Autodesk Inventor part; units mm, degrees
ref_plane "YZ Plane" through (0, 0, 0) normal (1, 0, 0) x (0, 1, 0)
ref_plane "XZ Plane" through (0, 0, 0) normal (0, 1, 0) x (-1, 0, 0)
ref_plane "XY Plane" through (0, 0, 0) normal (0, 0, 1) x (1, 0, 0)
sketch "スケッチ1" plane through (0, 0, 0) normal (0, 1, 0) x (-1, 0, 0)
  line L0 (-27.5, -9.5) -> (27.5, -9.5)
  line L1 (27.5, -9.5) -> (27.5, 9.5)
  line L2 (27.5, 9.5) -> (-27.5, 9.5)
  line L3 (-27.5, 9.5) -> (-27.5, -9.5)
  line L4 (-27.5, -9.5) -> (27.5, 9.5) construction
  line L5 (27.5, -9.5) -> (-27.5, 9.5) construction
  point P0 (0, 0)
  dimension "d0" = 19
  dimension "d1" = 55
extrude "プレート1" add sketch "スケッチ1" along normal blind 2
sketch "スケッチ2" plane through (27.5, 0, 9.5) normal (1, 0, 0) x (0, 0, -1)
  line L0 (0, 2) -> (19, 2)
  line L1 (19, 2) -> (0, 2)
  line L2 (0, 2) -> (0, 22)
  line L3 (0, 22) -> (19, 22)
  line L4 (19, 22) -> (19, 2)
  point P0 (9.5, 0)
  dimension "d3" = 20
sheet face with bend "面2" sketch "スケッチ2" thickness 2 toward (1, 0, 0) bend radius 2
bend "曲げ1"
sketch "スケッチ3" plane through (-27.5, 0, -9.5) normal (-1, 0, 0) x (0, 0, 1)
  line L0 (0, 0) -> (0, 2)
  line L1 (0, 22) -> (19, 22)
  line L2 (0, 2) -> (19, 2)
  line L3 (19, 2) -> (19, 22)
  line L4 (19, 22) -> (0, 22)
  line L5 (0, 22) -> (0, 2)
  point P0 (9.5, 0)
sheet face with bend "面3" sketch "スケッチ3" thickness 2 toward (-1, 0, 0) bend radius 2
bend "曲げ2"
sketch "スケッチ4" plane through (-29.5, 0, -9.5) normal (-1, 0, 0) x (0, 0, 1)
  line L0 (7.5, 18) -> (7.5, 8)
  arc A0 (7.5, 8) -> (11.5, 8) centre (9.5, 8) ccw
  line L1 (11.5, 8) -> (11.5, 18)
  arc A1 (11.5, 18) -> (7.5, 18) centre (9.5, 18) ccw
  line L2 (19, 22) -> (19, 4)
  line L3 (0, 22) -> (19, 22)
  line L4 (19, 4) -> (0, 4)
  point P0 (9.5, 0)
  dimension "d18" = 2
  dimension "d33" = 4
  dimension "d34" = 4
extrude "押し出し1" cut sketch "スケッチ4" against normal blind 100
sketch "スケッチ5" plane through (0, 2, 0) normal (0, 1, 0) x (1, 0, 0)
  line L0 (-19.5, -2) -> (19.5, -2)
  arc A0 (19.5, -2) -> (19.5, 2) centre (19.5, 0) ccw
  line L1 (19.5, 2) -> (-19.5, 2)
  arc A1 (-19.5, 2) -> (-19.5, -2) centre (-19.5, 0) ccw
  line L2 (25.5, -9.5) -> (-25.5, -9.5)
  line L3 (-25.5, 9.5) -> (-25.5, -9.5)
  line L4 (25.5, -9.5) -> (25.5, 9.5)
  point P0 (0, 0)
  point P1 (-21.5, 0)
  dimension "d22" = 2
  dimension "d35" = 6
  dimension "d36" = 6
extrude "押し出し2" cut sketch "スケッチ5" against normal blind 3
equation "\"d2\" = Thickness"
equation "\"d4\" = BendRadius"
equation "\"d5\" = BendReliefWidth"
equation "\"d7\" = MinimumRemnant"
equation "\"d6\" = BendReliefDepth"
equation "\"d8\" = TransitionRadius"
equation "\"d9\" = BendRadius"
equation "\"d10\" = BendReliefWidth"
equation "\"d12\" = MinimumRemnant"
equation "\"d11\" = BendReliefDepth"
equation "\"d13\" = TransitionRadius"
equation "\"BendRadius\" = Thickness"
equation "\"BendReliefWidth\" = Thickness"
equation "\"BendReliefDepth\" = 0.5 * Thickness"
equation "\"CornerReliefSize\" = 4 * Thickness"
equation "\"MinimumRemnant\" = 2 * Thickness"
equation "\"TransitionRadius\" = BendRadius"
equation "\"JacobiRadiusSize\" = BendRadius"
equation "\"GapSize\" = Thickness"
properties part number "thumbkey_cup" material "アルミニウム 6061"
The model under review builds one solid part; all positions refer to its coordinate system, in mm. A direction names the side the tool comes from. Give positions to 0.01 mm unless a question says otherwise; leave off trailing zeros. Write each loop counter-clockwise with the first axis right and the second up, starting at its lowest first coordinate (ties: lowest second). Pieces come first, ordered by that corner, then holes. Notation, with made-up numbers: (23.25, 66.5) - (38.25, 66.5) arc R19 cw to (38.25, 76.5) - close; hole circle Ø3 at (67.25, -36). An arc over 180 degrees is marked (long way). Answer in a Markdown table with one row per item. Add a question column.
1. Draft analysis for pull direction Y (two halves, no side actions). For faces 1 (the flat face through (0, 1, 2)), 2 (the cylindrical face through (28, 20, 0)), 3 (the flat face through (28, 22, 0)), 4 (the cylindrical face through (28, 6, 0)), state which applies: +Y half, -Y half, draft (parallel to the pull), parting line (faces both ways), or undercut.
2. Wall thickness on line 1 along X through (y, z) = (6, 4.25); line 2 along Y through (x, z) = (-22.5, -4.5); line 3 along X through (y, z) = (2.75, 3.5): over which ranges is each line inside the solid? List them lowest first. Write a range as [from, to].
3. We need section D-D on y = 17. Write out the cut boundary in (x, z).
4. We need section B-B on z = 0. Write out the cut boundary in (x, y), then the cut area to 3 significant figures.
5. Tool access review of faces 5 (the flat face through (0.1, 0.4, -9.5)), 6 (the cylindrical face through (-21.5, 1, 0)), 7 (the cylindrical face through (-29, 6, 0)), 8 (the cylindrical face through (26.93, 2.6, -0.13)): name each direction out of +Z, -Z, +X, -X, +Y, -Y from which nothing blocks a thin tool from reaching the whole face with its end or side.
6. We need section C-C on x = 3.5. Write out the cut boundary in (y, z).
7. We need section A-A on y = 4.75. Write out the cut boundary in (x, z), then the cut area to 3 significant figures.
8. Insertion check: P1, Ø3, axis at x = -14, z = -2.5, coming from the +Y side; P2, Ø9, axis at y = 10.5, z = -1, coming from the +X side. Each pin has a flat end and moves straight along its axis. Give the tip position at first contact, or say it passes through.
Ans:
| question | item | result |
|---|---|---|
| 1 | face 1 | draft |
| 1 | face 2 | undercut |
| 1 | face 3 | +Y half |
| 1 | face 4 | undercut |
| 2 | line 1 | x = [-29.5, -27.5], [27.5, 29.5] |
| 2 | line 2 | y = [0, 2] |
| 2 | line 3 | x = [-29.3, -27.06], [27.06, 29.3] |
| 3 | outline | (-29.5, -9.5) - (-27.5, -9.5) - (-27.5, -2) - (-29.5, -2) - close; (-29.5, 2) - (-27.5, 2) - (-27.5, 9.5) - (-29.5, 9.5) - close; (27.5, -9.5) - (29.5, -9.5) - (29.5, -2) - (27.5, -2) - close; (27.5, 2) - (29.5, 2) - (29.5, 9.5) - (27.5, 9.5) - close |
| 4 | outline | (-29.5, 4) arc R4 ccw to (-25.5, 0) - (-21.5, 0) - (-21.5, 2) - (-25.5, 2) arc R2 cw to (-27.5, 4) - (-27.5, 6) - (-29.5, 6) - close; (-29.5, 20) - (-27.5, 20) - (-27.5, 22) - (-29.5, 22) - close; (21.5, 0) - (25.5, 0) arc R4 ccw to (29.5, 4) - (29.5, 6) - (27.5, 6) - (27.5, 4) arc R2 cw to (25.5, 2) - (21.5, 2) - close; (27.5, 20) - (29.5, 20) - (29.5, 22) - (27.5, 22) - close |
| 4 | area | 50.8 mm^2 |
| 5 | face 5 | -Z, +X, -X, +Y, -Y |
| 5 | face 6 | +Y, -Y |
| 5 | face 7 | +X, -X |
| 5 | face 8 | +Z, -Z, +Y |
| 6 | outline | (0, -9.5) - (2, -9.5) - (2, -2) - (0, -2) - close; (0, 2) - (2, 2) - (2, 9.5) - (0, 9.5) - close |
| 7 | outline | (-29.5, -9.5) - (-27.5, -9.5) - (-27.5, 9.5) - (-29.5, 9.5) - close; (27.5, -9.5) - (29.5, -9.5) - (29.5, 9.5) - (27.5, 9.5) - close |
| 7 | area | 76.0 mm^2 |
| 8 | P1 | stops at y = 2 |
| 8 | P2 | stops at x = 29.5 |
